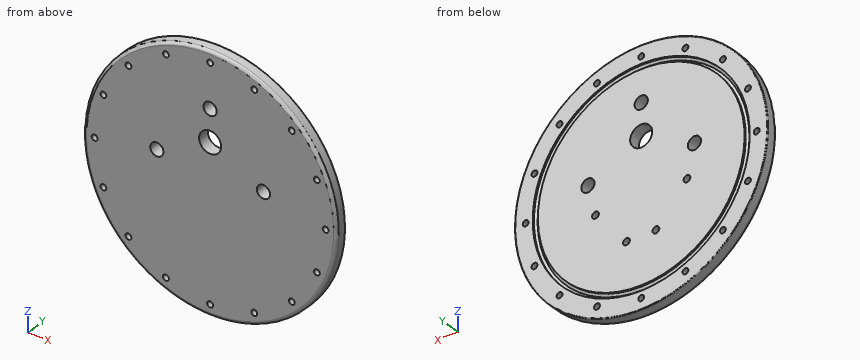
from build123d import *

# Parameters (mm, degrees)
SKETCH1_R           = 86
BOSS_EXTRUDE1_DEPTH = 8
CUT_EXTRUDE1_REACH  = 123.885
SKETCH2_R           = 2
SKETCH6_R           = 2.3
CUT_EXTRUDE3_DEPTH  = 6
CUT_EXTRUDE4_REACH  = 123.885
SKETCH8_R           = 4.5
SKETCH8_R_2         = 7.5
FILLET1_R           = 2
FILLET2_R           = 0.5


with BuildPart() as part:
    # Sketch1 → Boss-Extrude1 (new body)
    with BuildSketch(Plane(origin=(0, 0, 0), x_dir=(1, 0, 0), z_dir=(0, 1, 0))):
        with Locations(Location((0, 0, 0), (0, 0, 270))):
            Circle(SKETCH1_R)
    extrude(amount=BOSS_EXTRUDE1_DEPTH)

    # Sketch2 → Cut-Extrude1 (cut, up to next)
    with BuildSketch(Plane(origin=(0, 8, 0), x_dir=(1, 0, 0), z_dir=(0, 1, 0)), mode=Mode.PRIVATE) as cut_extrude1_sk1:
        with Locations(Location((0, 78.5, 0), (0, 0, 270))):
            Circle(SKETCH2_R)
    cut_extrude1_tool1 = extrude(cut_extrude1_sk1.sketch, amount=-CUT_EXTRUDE1_REACH, mode=Mode.PRIVATE) & part.part
    # Sketch2 → Cut-Extrude1 (cut, up to next)
    with BuildSketch(Plane(origin=(0, 8, 0), x_dir=(1, 0, 0), z_dir=(0, 1, 0)), mode=Mode.PRIVATE) as cut_extrude1_sk2:
        with Locations(Location((30.040649441, 72.524543302, 0), (0, 0, 270))):
            Circle(SKETCH2_R)
    cut_extrude1_tool2 = extrude(cut_extrude1_sk2.sketch, amount=-CUT_EXTRUDE1_REACH, mode=Mode.PRIVATE) & part.part
    # Sketch2 → Cut-Extrude1 (cut, up to next)
    with BuildSketch(Plane(origin=(0, 8, 0), x_dir=(1, 0, 0), z_dir=(0, 1, 0)), mode=Mode.PRIVATE) as cut_extrude1_sk3:
        with Locations(Location((55.507882323, 55.507882323, 0), (0, 0, 270))):
            Circle(SKETCH2_R)
    cut_extrude1_tool3 = extrude(cut_extrude1_sk3.sketch, amount=-CUT_EXTRUDE1_REACH, mode=Mode.PRIVATE) & part.part
    # Sketch2 → Cut-Extrude1 (cut, up to next)
    with BuildSketch(Plane(origin=(0, 8, 0), x_dir=(1, 0, 0), z_dir=(0, 1, 0)), mode=Mode.PRIVATE) as cut_extrude1_sk4:
        with Locations(Location((72.524543302, 30.040649441, 0), (0, 0, 270))):
            Circle(SKETCH2_R)
    cut_extrude1_tool4 = extrude(cut_extrude1_sk4.sketch, amount=-CUT_EXTRUDE1_REACH, mode=Mode.PRIVATE) & part.part
    # Sketch2 → Cut-Extrude1 (cut, up to next)
    with BuildSketch(Plane(origin=(0, 8, 0), x_dir=(1, 0, 0), z_dir=(0, 1, 0)), mode=Mode.PRIVATE) as cut_extrude1_sk5:
        with Locations(Location((78.5, 0, 0), (0, 0, 270))):
            Circle(SKETCH2_R)
    cut_extrude1_tool5 = extrude(cut_extrude1_sk5.sketch, amount=-CUT_EXTRUDE1_REACH, mode=Mode.PRIVATE) & part.part
    # Sketch2 → Cut-Extrude1 (cut, up to next)
    with BuildSketch(Plane(origin=(0, 8, 0), x_dir=(1, 0, 0), z_dir=(0, 1, 0)), mode=Mode.PRIVATE) as cut_extrude1_sk6:
        with Locations(Location((72.524543302, -30.040649441, 0), (0, 0, 270))):
            Circle(SKETCH2_R)
    cut_extrude1_tool6 = extrude(cut_extrude1_sk6.sketch, amount=-CUT_EXTRUDE1_REACH, mode=Mode.PRIVATE) & part.part
    # Sketch2 → Cut-Extrude1 (cut, up to next)
    with BuildSketch(Plane(origin=(0, 8, 0), x_dir=(1, 0, 0), z_dir=(0, 1, 0)), mode=Mode.PRIVATE) as cut_extrude1_sk7:
        with Locations(Location((55.507882323, -55.507882323, 0), (0, 0, 270))):
            Circle(SKETCH2_R)
    cut_extrude1_tool7 = extrude(cut_extrude1_sk7.sketch, amount=-CUT_EXTRUDE1_REACH, mode=Mode.PRIVATE) & part.part
    # Sketch2 → Cut-Extrude1 (cut, up to next)
    with BuildSketch(Plane(origin=(0, 8, 0), x_dir=(1, 0, 0), z_dir=(0, 1, 0)), mode=Mode.PRIVATE) as cut_extrude1_sk8:
        with Locations(Location((30.040649441, -72.524543302, 0), (0, 0, 270))):
            Circle(SKETCH2_R)
    cut_extrude1_tool8 = extrude(cut_extrude1_sk8.sketch, amount=-CUT_EXTRUDE1_REACH, mode=Mode.PRIVATE) & part.part
    # Sketch2 → Cut-Extrude1 (cut, up to next)
    with BuildSketch(Plane(origin=(0, 8, 0), x_dir=(1, 0, 0), z_dir=(0, 1, 0)), mode=Mode.PRIVATE) as cut_extrude1_sk9:
        with Locations(Location((0, -78.5, 0), (0, 0, 270))):
            Circle(SKETCH2_R)
    cut_extrude1_tool9 = extrude(cut_extrude1_sk9.sketch, amount=-CUT_EXTRUDE1_REACH, mode=Mode.PRIVATE) & part.part
    # Sketch2 → Cut-Extrude1 (cut, up to next)
    with BuildSketch(Plane(origin=(0, 8, 0), x_dir=(1, 0, 0), z_dir=(0, 1, 0)), mode=Mode.PRIVATE) as cut_extrude1_sk10:
        with Locations(Location((-30.040649441, -72.524543302, 0), (0, 0, 270))):
            Circle(SKETCH2_R)
    cut_extrude1_tool10 = extrude(cut_extrude1_sk10.sketch, amount=-CUT_EXTRUDE1_REACH, mode=Mode.PRIVATE) & part.part
    # Sketch2 → Cut-Extrude1 (cut, up to next)
    with BuildSketch(Plane(origin=(0, 8, 0), x_dir=(1, 0, 0), z_dir=(0, 1, 0)), mode=Mode.PRIVATE) as cut_extrude1_sk11:
        with Locations(Location((-55.507882323, -55.507882323, 0), (0, 0, 270))):
            Circle(SKETCH2_R)
    cut_extrude1_tool11 = extrude(cut_extrude1_sk11.sketch, amount=-CUT_EXTRUDE1_REACH, mode=Mode.PRIVATE) & part.part
    # Sketch2 → Cut-Extrude1 (cut, up to next)
    with BuildSketch(Plane(origin=(0, 8, 0), x_dir=(1, 0, 0), z_dir=(0, 1, 0)), mode=Mode.PRIVATE) as cut_extrude1_sk12:
        with Locations(Location((-72.524543302, -30.040649441, 0), (0, 0, 270))):
            Circle(SKETCH2_R)
    cut_extrude1_tool12 = extrude(cut_extrude1_sk12.sketch, amount=-CUT_EXTRUDE1_REACH, mode=Mode.PRIVATE) & part.part
    # Sketch2 → Cut-Extrude1 (cut, up to next)
    with BuildSketch(Plane(origin=(0, 8, 0), x_dir=(1, 0, 0), z_dir=(0, 1, 0)), mode=Mode.PRIVATE) as cut_extrude1_sk13:
        with Locations(Location((-78.5, 0, 0), (0, 0, 270))):
            Circle(SKETCH2_R)
    cut_extrude1_tool13 = extrude(cut_extrude1_sk13.sketch, amount=-CUT_EXTRUDE1_REACH, mode=Mode.PRIVATE) & part.part
    # Sketch2 → Cut-Extrude1 (cut, up to next)
    with BuildSketch(Plane(origin=(0, 8, 0), x_dir=(1, 0, 0), z_dir=(0, 1, 0)), mode=Mode.PRIVATE) as cut_extrude1_sk14:
        with Locations(Location((-72.524543302, 30.040649441, 0), (0, 0, 270))):
            Circle(SKETCH2_R)
    cut_extrude1_tool14 = extrude(cut_extrude1_sk14.sketch, amount=-CUT_EXTRUDE1_REACH, mode=Mode.PRIVATE) & part.part
    # Sketch2 → Cut-Extrude1 (cut, up to next)
    with BuildSketch(Plane(origin=(0, 8, 0), x_dir=(1, 0, 0), z_dir=(0, 1, 0)), mode=Mode.PRIVATE) as cut_extrude1_sk15:
        with Locations(Location((-55.507882323, 55.507882323, 0), (0, 0, 270))):
            Circle(SKETCH2_R)
    cut_extrude1_tool15 = extrude(cut_extrude1_sk15.sketch, amount=-CUT_EXTRUDE1_REACH, mode=Mode.PRIVATE) & part.part
    # Sketch2 → Cut-Extrude1 (cut, up to next)
    with BuildSketch(Plane(origin=(0, 8, 0), x_dir=(1, 0, 0), z_dir=(0, 1, 0)), mode=Mode.PRIVATE) as cut_extrude1_sk16:
        with Locations(Location((-30.040649441, 72.524543302, 0), (0, 0, 270))):
            Circle(SKETCH2_R)
    cut_extrude1_tool16 = extrude(cut_extrude1_sk16.sketch, amount=-CUT_EXTRUDE1_REACH, mode=Mode.PRIVATE) & part.part
    add(cut_extrude1_tool1.solids().sort_by_distance((0, 8, -78.5))[0], mode=Mode.SUBTRACT)
    add(cut_extrude1_tool2.solids().sort_by_distance((30.040649, 8, -72.524543))[0], mode=Mode.SUBTRACT)
    add(cut_extrude1_tool3.solids().sort_by_distance((55.507882, 8, -55.507882))[0], mode=Mode.SUBTRACT)
    add(cut_extrude1_tool4.solids().sort_by_distance((72.524543, 8, -30.040649))[0], mode=Mode.SUBTRACT)
    add(cut_extrude1_tool5.solids().sort_by_distance((78.5, 8, 0))[0], mode=Mode.SUBTRACT)
    add(cut_extrude1_tool6.solids().sort_by_distance((72.524543, 8, 30.040649))[0], mode=Mode.SUBTRACT)
    add(cut_extrude1_tool7.solids().sort_by_distance((55.507882, 8, 55.507882))[0], mode=Mode.SUBTRACT)
    add(cut_extrude1_tool8.solids().sort_by_distance((30.040649, 8, 72.524543))[0], mode=Mode.SUBTRACT)
    add(cut_extrude1_tool9.solids().sort_by_distance((0, 8, 78.5))[0], mode=Mode.SUBTRACT)
    add(cut_extrude1_tool10.solids().sort_by_distance((-30.040649, 8, 72.524543))[0], mode=Mode.SUBTRACT)
    add(cut_extrude1_tool11.solids().sort_by_distance((-55.507882, 8, 55.507882))[0], mode=Mode.SUBTRACT)
    add(cut_extrude1_tool12.solids().sort_by_distance((-72.524543, 8, 30.040649))[0], mode=Mode.SUBTRACT)
    add(cut_extrude1_tool13.solids().sort_by_distance((-78.5, 8, 0))[0], mode=Mode.SUBTRACT)
    add(cut_extrude1_tool14.solids().sort_by_distance((-72.524543, 8, -30.040649))[0], mode=Mode.SUBTRACT)
    add(cut_extrude1_tool15.solids().sort_by_distance((-55.507882, 8, -55.507882))[0], mode=Mode.SUBTRACT)
    add(cut_extrude1_tool16.solids().sort_by_distance((-30.040649, 8, -72.524543))[0], mode=Mode.SUBTRACT)

    # Sketch6 → Cut-Extrude3 (cut)
    with BuildSketch(Plane(origin=(0, 8, 0), x_dir=(1, 0, 0), z_dir=(0, 1, 0))):
        with Locations(Location((-10, 38, 0), (0, 0, 270))):
            Circle(SKETCH6_R)
        with Locations(Location((10, 38, 0), (0, 0, 270))):
            Circle(SKETCH6_R)
        with Locations(Location((-31.087993015, 12.771112084, 0), (0, 0, 270))):
            Circle(SKETCH6_R)
        with Locations(Location((31.092199918, 12.771112084, 0), (0, 0, 270))):
            Circle(SKETCH6_R)
    extrude(amount=-CUT_EXTRUDE3_DEPTH, mode=Mode.SUBTRACT)

    # Sketch8 → Cut-Extrude4 (cut, up to next)
    with BuildSketch(Plane(origin=(0, 8, 0), x_dir=(1, 0, 0), z_dir=(0, 1, 0)), mode=Mode.PRIVATE) as cut_extrude4_sk1:
        with Locations(Location((-36.2, -8.428843365, 0), (0, 0, 270))):
            Circle(SKETCH8_R)
    cut_extrude4_tool1 = extrude(cut_extrude4_sk1.sketch, amount=-CUT_EXTRUDE4_REACH, mode=Mode.PRIVATE) & part.part
    # Sketch8 → Cut-Extrude4 (cut, up to next)
    with BuildSketch(Plane(origin=(0, 8, 0), x_dir=(1, 0, 0), z_dir=(0, 1, 0)), mode=Mode.PRIVATE) as cut_extrude4_sk2:
        with Locations(Location((36.2, -8.428843365, 0), (0, 0, 270))):
            Circle(SKETCH8_R)
    cut_extrude4_tool2 = extrude(cut_extrude4_sk2.sketch, amount=-CUT_EXTRUDE4_REACH, mode=Mode.PRIVATE) & part.part
    # Sketch8 → Cut-Extrude4 (cut, up to next)
    with BuildSketch(Plane(origin=(0, 8, 0), x_dir=(1, 0, 0), z_dir=(0, 1, 0)), mode=Mode.PRIVATE) as cut_extrude4_sk3:
        with Locations(Location((0, -48.566515497, 0), (0, 0, 270))):
            Circle(SKETCH8_R)
    cut_extrude4_tool3 = extrude(cut_extrude4_sk3.sketch, amount=-CUT_EXTRUDE4_REACH, mode=Mode.PRIVATE) & part.part
    # Sketch8 → Cut-Extrude4 (cut, up to next)
    with BuildSketch(Plane(origin=(0, 8, 0), x_dir=(1, 0, 0), z_dir=(0, 1, 0)), mode=Mode.PRIVATE) as cut_extrude4_sk4:
        with Locations(Location((0, -26.826761031, 0), (0, 0, 270))):
            Circle(SKETCH8_R_2)
    cut_extrude4_tool4 = extrude(cut_extrude4_sk4.sketch, amount=-CUT_EXTRUDE4_REACH, mode=Mode.PRIVATE) & part.part
    add(cut_extrude4_tool1.solids().sort_by_distance((-36.2, 8, 8.428843))[0], mode=Mode.SUBTRACT)
    add(cut_extrude4_tool2.solids().sort_by_distance((36.2, 8, 8.428843))[0], mode=Mode.SUBTRACT)
    add(cut_extrude4_tool3.solids().sort_by_distance((0, 8, 48.566515))[0], mode=Mode.SUBTRACT)
    add(cut_extrude4_tool4.solids().sort_by_distance((0, 8, 26.826761))[0], mode=Mode.SUBTRACT)

    # Sketch4 → Cut-Revolve1 (revolve, cut)
    with BuildSketch(Plane.XY, mode=Mode.PRIVATE) as cut_revolve1_sk:
        Polygon((73.75, 6.880362971), (73.75, 8), (70.25, 8), (70.25, 6.880362971), (72, 5.87), align=None)
    revolve(cut_revolve1_sk.sketch.rotate(Axis((0, 0, 0), (0, 1, 0)), 90), axis=Axis((0, 0, 0), (0, 1, 0)), mode=Mode.SUBTRACT)

    # Fillet1
    fillet1_edges = [part.edges().sort_by_distance(p)[0] for p in [
        (0, 0, -86),
    ]]
    fillet(fillet1_edges, radius=FILLET1_R)

    # Fillet2
    fillet2_edges = [part.edges().sort_by_distance(p)[0] for p in [
        (0, 8, -86),
    ]]
    fillet(fillet2_edges, radius=FILLET2_R)


solid = part.part
Could you check a few things on this model? Use its own coordinates, in mm. Coordinates: 2 decimals unless noted, no trailing zeros. Write each loop counter-clockwise with the first axis right and the second up, starting at its lowest first coordinate (ties: lowest second). Pieces come first, ordered by that corner, then holes. Notation, with made-up numbers: M -2,-16 L 29,-16 A16 ccw 29,7 Z; hole C -27.75,1.5 d8. An arc over 180 degrees is marked long. One line per question, with ' | ' between items.
1) For pin 1 Ø3 at (x, y) = (6, 4) entering from +Z; pin 2 Ø1 at (x, y) = (55, 2.5) entering from -Z; pin 3 Ø1.4 at (x, z) = (-9, -38.5) entering from +Y, each with a flat end and sliding along its axis, tell me the tip position at first contact or that it passes through.
Checks:
pin 1: z = 85.88 | pin 2: z = -66.53 | pin 3: y = 2
2) Imagine slicing it at A-A, the plane z = 0. Write out the boundary of the cut face in (x, y).
Checks:
outline: M -86,2 A2 ccw -84,0 L -80.5,0 L -80.5,8 L -85.5,8 A0.5 ccw -86,7.5 Z; M -76.5,0 L 76.5,0 L 76.5,8 L 73.75,8 L 73.75,6.88 L 72,5.87 L 70.25,6.88 L 70.25,8 L -70.25,8 L -70.25,6.88 L -72,5.87 L -73.75,6.88 L -73.75,8 L -76.5,8 Z; M 80.5,0 L 84,0 A2 ccw 86,2 L 86,7.5 A0.5 ccw 85.5,8 L 80.5,8 Z
3) Imagine slicing it at B-B, the plane y = 4.5. Give the number of separate pieces and of enclosed holes in the cut face, and give its area (3 significant figures).
Checks:
separate pieces: 1 | enclosed holes: 24 | area: 22,600 mm²
4) I need wall thicknesses on probe 1 along X at (y, z) = (4.75, 0); probe 2 along X at (y, z) = (1.75, 71); probe 3 along X at (y, z) = (1, 31). Which ranges of each line are inside material? Lowest first, please. Write a range as [from, to].
Checks:
probe 1: [-86, -80.5], [-76.5, 76.5], [80.5, 86] | probe 2: [-48.5, -31.34], [-28.75, 28.75], [31.34, 48.5] | probe 3: [-79.93, -74.28], [-70.77, -6.23], [6.23, 70.77], [74.28, 79.93]
